The drawing under review shows one solid part. Ordinate dimensions are in mm from its lowest x, y, z. A direction names the side the tool comes from. Coordinates: 2 decimals unless noted, no trailing zeros. Order: outer loops, then holes, each group sorted by start corner. A loop starts at its lowest first (then second) coordinate and runs counter-clockwise, first axis right, second up.
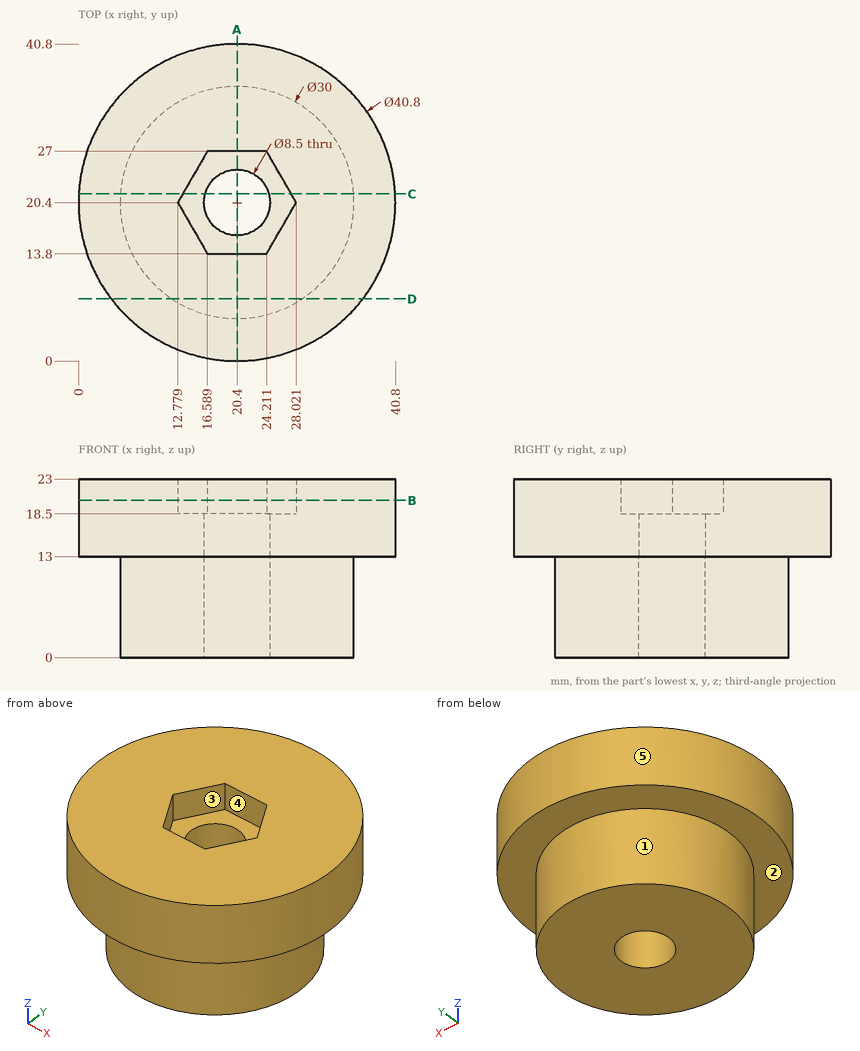
1. Take a section at A-A, the plane x = 20.4. Give the boundary of the cut face in (y, z).
Answer below:
outline: (0, 13) - (5.4, 13) - (5.4, 0) - (16.15, 0) - (16.15, 18.5) - (13.8, 18.5) - (13.8, 23) - (0, 23) - close; (24.65, 0) - (35.4, 0) - (35.4, 13) - (40.8, 13) - (40.8, 23) - (27, 23) - (27, 18.5) - (24.65, 18.5) - close
2. Take a section at C-C, the plane y = 21.5. Give the boundary of the cut face in (x, z) (1 decimal).
Answer below:
outline: (0, 13) - (5.4, 13) - (5.4, 0) - (16.3, 0) - (16.3, 18.5) - (13.4, 18.5) - (13.4, 23) - (0, 23) - close; (24.5, 0) - (35.4, 0) - (35.4, 13) - (40.8, 13) - (40.8, 23) - (27.4, 23) - (27.4, 18.5) - (24.5, 18.5) - close
3. To check wall thickness, follow L1, parallel to Y at x = 20.4, z = 6.5; L2, parallel to Z at x = 4, y = 13; L3, parallel to Y at x = 19, z = 7.75 (1 decimal). State the ranges of each line that lie inside material, in increasing order.
Answer below:
L1: y = 5.4 to 16.15, 24.65 to 35.4
L2: z = 13 to 23
L3: y = 5.5 to 16.4, 24.4 to 35.3
4. Take a section at D-D, the plane y = 8. Give the boundary of the cut face in (x, z).
Answer below:
outline: (4.2, 13) - (11.96, 13) - (11.96, 0) - (28.84, 0) - (28.84, 13) - (36.6, 13) - (36.6, 23) - (4.2, 23) - close
5. Take a section at B-B, the plane z = 20.25. Give the boundary of the cut face in (x, y), plus the area to 3 significant figures.
Answer below:
outline: circle Ø40.8 at (20.4, 20.4); hole (12.78, 20.4) - (16.59, 13.8) - (24.21, 13.8) - (28.02, 20.4) - (24.21, 27) - (16.59, 27) - close
area: 1,160 mm2
6. Machinability: for the marked faces 4 and 5, which of the approach directions +Z, -Z, +X, -X, +Y, -Y give a long, thin tool a straight path to every point of the face, cutting with its end or side? Answer none if there is none.
Answer below:
face 4: +Z
face 5: +Z, -Z
7. Clearance check with flat-ended pins moving along their axes: pin 1 Ø10 at (y, z) = (5.5, 5) entering from -X; pin 2 Ø5 at (y, z) = (4.5, 6) entering from +X; pin 3 Ø5 at (x, z) = (15.5, 9.5) entering from +Y; pin 4 Ø7.5 at (x, y) = (20.4, 20.4) entering from +Z. State where each tip first meets the part, or that it passes through.
Answer below:
pin 1: stops at x = 9.13
pin 2: stops at x = 27.14
pin 3: stops at y = 35.21
pin 4: passes through
8. The part is to be moulded in two halves that separate along Y. For the marked faces 1, 2 and 3, say which applies: +Y half, -Y half, draft (parallel to the pull), parting line (faces both ways), or undercut.
Answer below:
face 1: parting line
face 2: draft
face 3: undercut
